```python
from build123d import *

# Parameters (mm, degrees)
STEM_START                = -3.244746183
STEM_OTHER_SIDE_OUTLINE_W = 12.827
STEM_OTHER_SIDE_OUTLINE_H = 3.302
STEM_OTHER_SIDE_OUTLINE_R = 3.81
STEM_OTHER_SIDE_DEPTH     = 3.175
SKETCH1_R                 = 3.4925
CUT_EXTRUDE1_DEPTH        = 3.175


# Read off the part's stored shape, not the designer's step: Stem Other Side
with BuildPart() as part:
    # Stem Other Side outline → Stem Other Side (new body)
    with BuildSketch(Plane(origin=(0, 0, 0), x_dir=(1, 0, 0), z_dir=(0, 1, 0)).offset(STEM_START)):
        with BuildLine():
            Line((-4.25309824, 33.316184511), (-5.52309824, 33.316184511))
            ThreePointArc((-5.52309824, 33.316184511), (-11.809277525, 30.712363796), (-14.41309824, 24.426184511))
            Line((-14.41309824, 24.426184511), (-14.41309824, -42.883815489))
            Line((-14.41309824, -42.883815489), (4.63690176, -42.883815489))
            Line((4.63690176, -42.883815489), (4.63690176, 24.426184511))
            ThreePointArc((4.63690176, 24.426184511), (2.033081045, 30.712363796), (-4.25309824, 33.316184511))
        make_face()
        with Locations((-4.88809824, -12.784815489)):
            Rectangle(STEM_OTHER_SIDE_OUTLINE_W, STEM_OTHER_SIDE_OUTLINE_H, mode=Mode.SUBTRACT)
        with Locations((-4.88809824, 20.616184511)):
            Circle(STEM_OTHER_SIDE_OUTLINE_R, mode=Mode.SUBTRACT)
    extrude(amount=STEM_OTHER_SIDE_DEPTH)

    # Sketch1 → Cut-Extrude1 (cut)
    with BuildSketch(Plane(origin=(0, -0.069746183, 0), x_dir=(1, 0, 0), z_dir=(0, 1, 0))):
        with Locations(Location((-4.88809824, -36.533815489, 0), (0, 0, 270))):
            Circle(SKETCH1_R)
    extrude(amount=-CUT_EXTRUDE1_DEPTH, mode=Mode.SUBTRACT)


solid = part.part
```
The model under review builds one solid part; all positions refer to its coordinate system, in mm. A direction names the side the tool comes from. Round coordinates to 2 decimals unless told otherwise and drop trailing zeros. Loops run counter-clockwise (first coordinate to the right, second up) from the corner with the lowest first, then second, coordinate; pieces in that order, holes last. Notation, with made-up numbers: M 15.25,20.25 L 71.25,20.25 A13 cw 71.25,45.25 Z; hole C -8,18 d1. An arc over 180 degrees is marked long. Write item = value, one per line.
Item 1: Take a section at D-D on x = -12.25. Write out the cut boundary in (y, z), then the cut area to 3 significant figures.
Return value:
outline = M -3.24,-30.24 L -0.07,-30.24 L -0.07,42.88 L -3.24,42.88 Z
area = 232 mm2
Item 2: Take a section at A-A on z = 36. Write out the cut boundary in (x, y), then the cut area to 3 significant figures.
Return value:
outline = M -14.41,-3.24 L -8.34,-3.24 L -8.34,-0.07 L -14.41,-0.07 Z; M -1.44,-3.24 L 4.64,-3.24 L 4.64,-0.07 L -1.44,-0.07 Z
area = 38.6 mm2
Item 3: The part is to be moulded in two halves that separate along X. For faces 3 (the flat face through (-14.413, -2, 9)), 4 (the flat face through (-5, -2, -33.316)), 5 (the flat face through (1.525, -2, 13)), 6 (the flat face through (4.637, -2, 10)), say which applies: released by +X, released by -X, zero draft, split by the parting line, or undercut.
Return value:
face_3 = released by -X
face_4 = zero draft
face_5 = undercut
face_6 = released by +X
Item 4: Take a section at C-C on y = -1.7. Write out the cut boundary in (x, z) (1 decimal).
Return value:
outline = M -14.4,-24.4 A8.9 ccw -5.5,-33.3 L -4.3,-33.3 A8.9 ccw 4.6,-24.4 L 4.6,42.9 L -14.4,42.9 Z; hole M -11.3,11.1 L 1.5,11.1 L 1.5,14.4 L -11.3,14.4 Z; hole C -4.9,-20.6 d7.6; hole C -4.9,36.5 d7
Item 5: Machinability: for faces 1 (the flat face through (-5, -3.245, 4)), 2 (the flat face through (-5, -2, 11.134)), which of the approach directions +Z, -Z, +X, -X, +Y, -Y give a long, thin tool a straight path to every point of the face, cutting with its end or side? Answer none if there is none.
Return value:
face_1 = +Z, -Z, +X, -X, -Y
face_2 = +Y, -Y
Item 6: Take a section at B-B on x = -7.25. Write out the cut boundary in (y, z).
Return value:
outline = M -3.24,-33.15 L -0.07,-33.15 L -0.07,-23.61 L -3.24,-23.61 Z; M -3.24,-17.63 L -0.07,-17.63 L -0.07,11.13 L -3.24,11.13 Z; M -3.24,14.44 L -0.07,14.44 L -0.07,33.96 L -3.24,33.96 Z; M -3.24,39.11 L -0.07,39.11 L -0.07,42.88 L -3.24,42.88 Z
Item 7: For line 1 (Z direction, x = -1.75, y = -1.8); line 2 (X direction, y = -1.6, z = 37); line 3 (X direction, y = -0.75, z = -23), list the stretches that pass through material, from the lowest coordinate up. Write a range as [from, to].
Return value:
line_1 = [-32.96, -22.78], [-18.46, 11.13], [14.44, 35], [38.07, 42.88]
line_2 = [-14.41, -8.35], [-1.43, 4.64]
line_3 = [-14.41, -7.86], [-1.92, 4.64]
